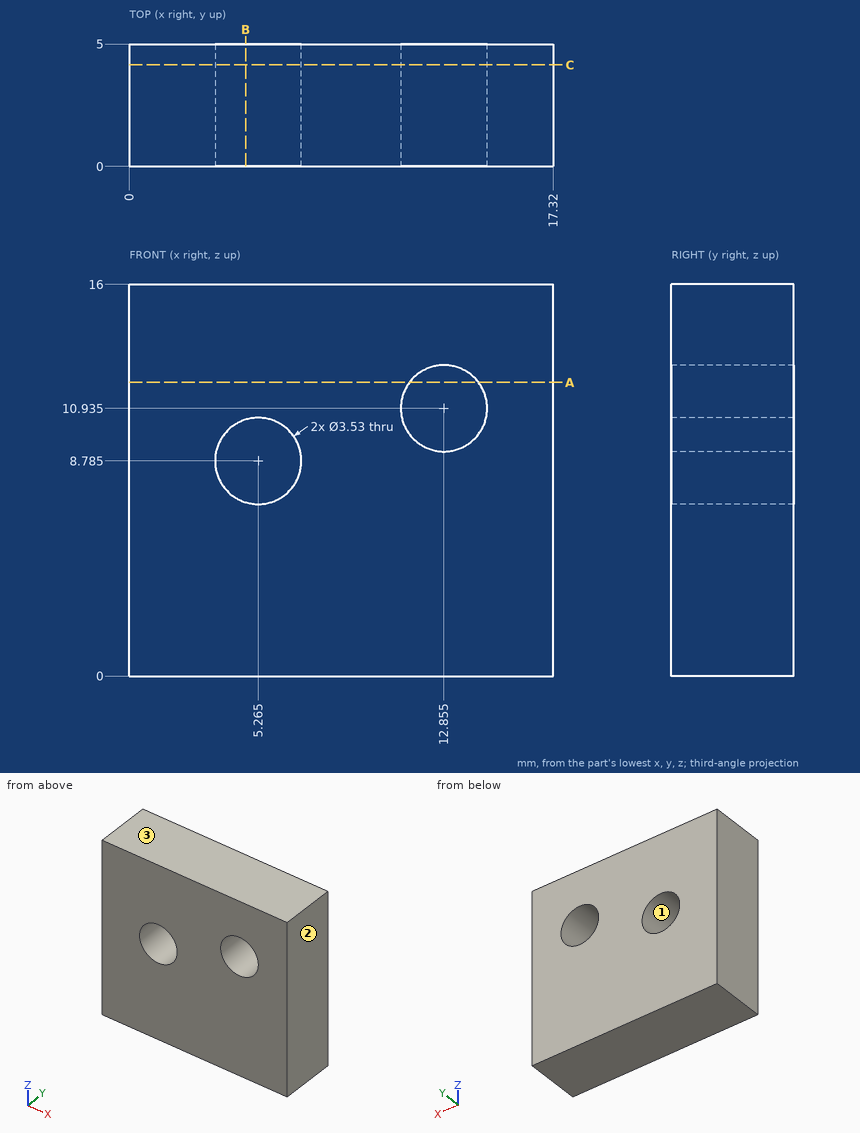
Could you check a few things on this drawing? It's one solid part, dimensions in mm from its lowest x, y, z. Round coordinates to 2 decimals unless told otherwise and drop trailing zeros. Order: outer loops, then holes, each group sorted by start corner. A loop starts at its lowest first (then second) coordinate and runs counter-clockwise, first axis right, second up. Notation, with made-up numbers: M 19.5,-3.75 L 61.5,-3.75 A22 ccw 61.5,31.25 Z; hole C -20.75,19 d8. An arc over 180 degrees is marked long. One line per question, with ' | ' between items.
1) We'd pull the mould along Z, two halves only. Please class the marked faces 1, 2 and 3: released by +Z, released by -Z, zero draft, split by the parting line, or undercut.
Checked values:
face 1: undercut | face 2: zero draft | face 3: released by +Z
2) Imagine slicing it at B-B, the plane x = 4.75. Write out the boundary of the cut face in (y, z), plus the area to 3 significant figures.
Checked values:
outline: M 0,0 L 5,0 L 5,7.1 L 0,7.1 Z; M 0,10.47 L 5,10.47 L 5,16 L 0,16 Z | area: 63.1 mm²
3) I need wall thicknesses on line 1 (Z direction, x = 12.75, y = 2.65); line 2 (Z direction, x = 11.5, y = 3.3); line 3 (X direction, y = 0.45, z = 8). Which ranges of each line are inside material? Lowest first, please.
Checked values:
line 1: z = 0 to 9.17, 12.7 to 16 | line 2: z = 0 to 9.8, 12.07 to 16 | line 3: x = 0 to 3.68, 6.85 to 17.32
4) Imagine slicing it at C-C, the plane y = 4.15. Write out the boundary of the cut face in (x, z) (3 decimals).
Checked values:
outline: M 0,0 L 17.32,0 L 17.32,16 L 0,16 Z; hole C 5.265,8.785 d3.53; hole C 12.855,10.935 d3.53
5) Imagine slicing it at A-A, the plane z = 12. Write out the boundary of the cut face in (x, y).
Checked values:
outline: M 0,0 L 11.45,0 L 11.45,5 L 0,5 Z; M 14.26,0 L 17.32,0 L 17.32,5 L 14.26,5 Z
